Work out the finished part from the listing and answer in its coordinate system (mm). Face numbers are marked on the shaded views. A direction names the side the tool comes from. Give positions to 0.01 mm unless a question says otherwise; leave off trailing zeros. Order: outer loops, then holes, each group sorted by start corner. A loop starts at its lowest first (then second) coordinate and runs counter-clockwise, first axis right, second up. Notation, with made-up numbers: (56.5, 82.5) -> (97.5, 82.5) arc R24 cw to (97.5, 99.5) -> close; hole circle Ø7 at (13, -22.5). An arc over 180 degrees is marked (long way). Use a Markdown table: item, result. Add a question column.
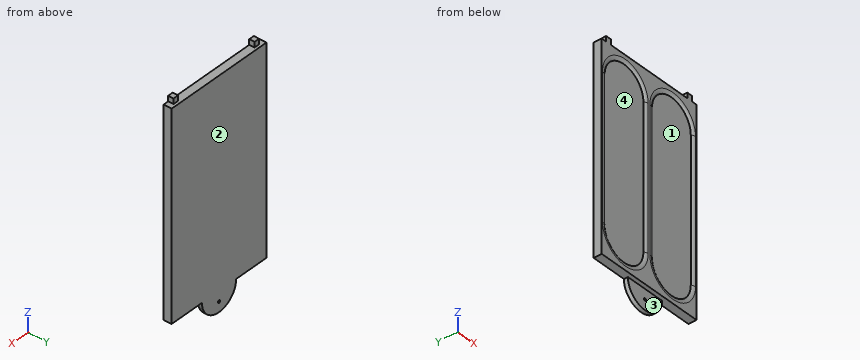
Autodesk Inventor part; units mm, degrees
ref_plane "YZ Plane" through (0, 0, 0) normal (1, 0, 0) x (0, 1, 0)
ref_plane "XZ Plane" through (0, 0, 0) normal (0, 1, 0) x (-1, 0, 0)
ref_plane "XY Plane" through (0, 0, 0) normal (0, 0, 1) x (1, 0, 0)
sketch "Sketch1" plane through (0, 0, 0) normal (0, 1, 0) x (-1, 0, 0)
  line L0 (0, 0) -> (41.5, 0)
  line L1 (41.5, 0) -> (41.5, -76)
  line L2 (41.5, -76) -> (0, -76)
  line L3 (0, -76) -> (0, 0)
  dimension "d0" = 41.5
  dimension "d1" = 76
extrude "Extrusion1" add sketch "Sketch1" along normal blind 3
sketch "Sketch2" plane through (-41.5, 0, 0) normal (0, 0, 1) x (1, 0, 0)
  line L0 (41.5, 0) -> (0, 0) construction
  line L1 (0, 0) -> (2, 0) construction
  line L2 (41.5, 0) -> (41.5, 3) construction
  line L3 (41.5, 0) -> (39.5, 0) construction
  line L4 (2, 0) -> (4, 0)
  line L5 (4, 0) -> (4, 2)
  line L6 (4, 2) -> (2, 2)
  line L7 (2, 2) -> (2, 0)
  line L8 (39.5, 0) -> (37.5, 0)
  line L9 (37.5, 0) -> (37.5, 2)
  line L10 (37.5, 2) -> (39.5, 2)
  line L11 (39.5, 2) -> (39.5, 0)
  dimension "d4" = 2
  dimension "d5" = 2
  dimension "d6" = 2
  dimension "d7" = 2
  dimension "d8" = 2
  dimension "d9" = 2
extrude "Extrusion2" add sketch "Sketch2" along normal blind 2
sketch "Sketch3" plane through (0, 3, 0) normal (0, 1, 0) x (1, 0, 0)
  line L0 (0, 76) -> (-41.5, 76)
  circle A0 centre (-20.75, 76) radius 7.5
  point P0 (0, 0)
  point P1 (-28.25, 76)
  point P2 (-13.25, 76)
  dimension "d12" = 15
extrude "Extrusion3" add sketch "Sketch3" against normal blind 1.5 contours L0 A0 picked at (-18.3226, 76.5983)
sketch "Sketch4" plane through (0, 3, 0) normal (0, 1, 0) x (1, 0, 0)
  line L0 (-28.25, 76) -> (-13.25, 76) construction
  line L1 (-20.75, 76) -> (-20.75, 79.75) construction
  point P0 (0, 0)
  dimension "d15" = 3.75
hole "Hole1" at (-20.75, 3, -79.75) direction (0, -1, 0) diameter 1 depth 2 tip angle 118
sketch "Sketch5" plane through (0, 0, 0) normal (0, -1, 0) x (1, 0, 0)
  line L0 (-28.25, -76) -> (-13.25, -76) construction
  line L1 (-20.75, -76) -> (-20.75, 0) construction
  line L2 (-41.5, 0) -> (0, 0) construction
  line L3 (-41.5, -76) -> (-41.5, 0) construction
  line L4 (-41.5, -76) -> (-20.75, 0) construction
  line L5 (-41.5, 0) -> (-20.75, -76) construction
  line L6 (-28.25, -76) -> (-41.5, -76) construction
  line L7 (-31.125, -76) -> (-31.125, -73) construction
  line L8 (-31.125, 0) -> (-31.125, -3) construction
  line L9 (-31.125, -73) -> (-31.125, -3) construction
  line L10 (-22.625, -64.5) -> (-22.625, -11.5)
  line L11 (-39.625, -11.5) -> (-39.625, -64.5)
  arc A0 (-39.625, -64.5) -> (-22.625, -64.5) centre (-31.125, -64.5) ccw
  arc A1 (-22.625, -11.5) -> (-39.625, -11.5) centre (-31.125, -11.5) ccw
  line L12 (-18.875, -64.5) -> (-18.875, -11.5)
  line L13 (-1.875, -11.5) -> (-1.875, -64.5)
  arc A2 (-18.875, -64.5) -> (-1.875, -64.5) centre (-10.375, -64.5) ccw
  arc A3 (-1.875, -11.5) -> (-18.875, -11.5) centre (-10.375, -11.5) ccw
  point P0 (-31.125, -38)
  dimension "d23" = 3
  dimension "d24" = 3
  dimension "d25" = 17
extrude "Extrusion4" cut sketch "Sketch5" against normal blind 0.5
fillet "Fillet1" radius 2.5 8 edges at (-31.125, 0, -73) (-39.625, 0, -38) (-31.125, 0, -3) (-22.625, 0, -38) (-10.375, 0, -3) (-1.875, 0, -38) (-10.375, 0, -73) (-18.875, 0, -38)
properties part number "tapa pila"
1) Straight lines are drawn through the part: line 1 (Z direction, x = -20.75, y = 2.05); line 2 (X direction, y = 0.2, z = -29); line 3 (Y direction, x = -36, z = -43). For each, find the intervals that lie inside material, in ascending order.
2) Which of the six approach directions +Z, -Z, +X, -X, +Y, -Y give full straight-line access (tool end or side, diameter ignored) to the marked faces 1 and 2?
3) Determine the mould class of the marked faces 3 and 4 for opening direction Z: released by +Z, released by -Z, zero draft, split by the parting line, or undercut.
4) Flat-ended cylindrical pins translate along their axes: pin 1 (1.5 mm diameter, centred on x = -8.5, z = -45.5, fed in from -Y); pin 2 (0.6 mm diameter, centred on y = 1, z = 1, fed in from -X); pin 3 (1.6 mm diameter, centred on y = 0.5, z = 0.5, fed in from +X); pin 4 (1.6 mm diameter, centred on x = -39, z = 1, fed in from +Y). Find the tip coordinate at first contact, or state that the pin passes through.
5) The part is cut by section A-A, the plane z = -30. Determine the outline of the cut face in (x, y) (3 decimals), then the cut area to 3 significant figures.
A:
| question | item | result |
|---|---|---|
| 1 | line 1 | -83.5 to -80.25, -79.25 to 0 |
| 1 | line 2 | -41.5 to -40.15, -22.1 to -19.4, -1.35 to 0 |
| 1 | line 3 | 0.5 to 3 |
| 2 | face 1 | -Y |
| 2 | face 2 | +Z, -Z, +X, -X, +Y |
| 3 | face 3 | zero draft |
| 3 | face 4 | undercut |
| 4 | pin 1 | y = 0.5 |
| 4 | pin 2 | x = -39.5 |
| 4 | pin 3 | x = 0 |
| 4 | pin 4 | y = 2 |
| 5 | outline | (-41.5, 0) -> (-41.125, 0) arc R2.5 ccw to (-39.625, 0.5) -> (-22.625, 0.5) arc R2.5 ccw to (-21.125, 0) -> (-20.375, 0) arc R2.5 ccw to (-18.875, 0.5) -> (-1.875, 0.5) arc R2.5 ccw to (-0.375, 0) -> (0, 0) -> (0, 3) -> (-41.5, 3) -> close |
| 5 | area | 107 mm^2 |
